Geometry: final body of the model. Coordinates: model frame, mm. A direction names the side the tool comes from. Round coordinates to 2 decimals unless told otherwise and drop trailing zeros. Write each loop counter-clockwise with the first axis right and the second up, starting at its lowest first coordinate (ties: lowest second). Pieces come first, ordered by that corner, then holes. Notation, with made-up numbers: M -2,-37 L 10,-37 A31 ccw 10,-8 Z; hole C 27.5,-37 d8. An arc over 180 degrees is marked long. Answer as CSV lines item,"result". Start each with the question number.
Q1. Section query A-A on z = 234. Output: boundary loops of the cut face in (x, y).
Q2. Section query C-C on y = 6. Output: boundary loops of the cut face in (x, z), and give its area (3 significant figures).
Q3. Mould query, pull axis Z, two halves, no side actions, for faces 1 (the flat face through (-151.164, -3, 200)), 2 (the flat face through (-40.966, -20.171, 17.605)), 3 (the flat face through (-110, -3, 147.99)), 4 (the flat face through (-151.164, -3, 277)). Classes: pulls with the +Z half, pulls with the -Z half, needs draft (parallel to the pull), parting line crosses it, or undercut.
Q4. First-contact query: pin 1 (4 mm diameter, centred on x = -59, y = -1, fed in from +Z); pin 2 (5 mm diameter, centred on x = -195, y = -4.5, fed in from -Z); pin 3 (12 mm diameter, centred on y = -10.5, z = 121.5, fed in from +X). Flat tips, straight axial feed; report the tip coordinate or a pass-through.
Q5. Reachability of faces 5 (the flat face through (-13.889, -5, 132)), 6 (the flat face through (-220.841, -3, 248)), 7 (the flat face through (-109, -3, 137.605)), 8 (the flat face through (-157, -8, 206)) from +Z, -Z, +X, -X, +Y, -Y: full face, straight path, thin tool, end or side. Return the list, or none.
Q6. Section query B-B on x = -89. Output: boundary loops of the cut face in (y, z).
Q7. Ray query, probe 1 along Z at (x, y) = (-183, -6); probe 2 along X at (y, z) = (1, 270.5); probe 3 along X at (y, z) = (-6, 216). Return the intervals inside material, ascending.
Q8. Section query D-D on z = 92.5. Output: boundary loops of the cut face in (x, y).
```python
from build123d import *

# Parameters (mm, degrees)
SKETCH_1_W      = 68.292893219
SKETCH_1_H      = 68.292893218
EXTRUDE_1_DEPTH = 10
SKETCH_2_W      = 53.40749746
SKETCH_2_H      = 14.776374923
EXTRUDE_2_DEPTH = 270
SKETCH_4_W      = 27.47748939
SKETCH_4_H      = 82.93676663
SKETCH_4_H_2    = 74.09911356
SKETCH_4_W_2    = 31.70911111
EXTRUDE_3_DEPTH = 10
CHAMFER_1_SIZE  = 15
CHAMFER_3_SIZE  = 7
FILLET_3_R      = 5
CHAMFER_4_SIZE  = 4


with BuildPart() as part:
    # 草图1 → 凸台-拉伸1 (new body)
    with BuildSketch(Plane.XY):
        with Locations((-33.149855831, 2)):
            Rectangle(SKETCH_1_W, SKETCH_1_H)
    extrude(amount=EXTRUDE_1_DEPTH)

    # 草图2 → 凸台-拉伸2 (add)
    with BuildSketch(Plane.XY.offset(10)):
        with Locations((-40.59255371, -5.388187462)):
            Rectangle(SKETCH_2_W, SKETCH_2_H)
    extrude(amount=EXTRUDE_2_DEPTH)

    # 草图4 → 凸台-拉伸3 (add)
    with BuildSketch(Plane(origin=(0, 2, 0), x_dir=(1, 0, 0), z_dir=(0, 1, 0))):
        Polygon((-151.163737931, -260.803324395), (-67.29630244, -260.803324395), (-67.29630244, -249.935229756), (-151.163737931, -249.935229756), (-151.163737931, -147.989777894), (-67.29630244, -147.989777894), (-67.29630244, -137.604662475), (-151.163737931, -137.604662475), (-151.163737931, -117.751683705), (-229.082858204, -117.751683705), (-229.082858204, -294.217578605), (-151.163737931, -294.217578605), align=None)
        with Locations((-207.102608026, -247.45301447)):
            Rectangle(SKETCH_4_W, SKETCH_4_H, mode=Mode.SUBTRACT)
        with Locations((-207.102608026, -162.803209554)):
            Rectangle(SKETCH_4_W, SKETCH_4_H_2, mode=Mode.SUBTRACT)
        with Locations((-172.622136648, -247.45301447)):
            Rectangle(SKETCH_4_W_2, SKETCH_4_H, mode=Mode.SUBTRACT)
        with Locations((-172.622136648, -162.803209554)):
            Rectangle(SKETCH_4_W_2, SKETCH_4_H_2, mode=Mode.SUBTRACT)
    extrude(amount=-EXTRUDE_3_DEPTH)

    # 倒角1
    chamfer_1_edges = [part.edges().sort_by_distance(p)[0] for p in [
        (-40.59255371, 2, 10),
        (-40.59255371, -12.776374923, 10),
    ]]
    chamfer(chamfer_1_edges, length=CHAMFER_1_SIZE)

    # 倒角3
    chamfer_3_edges = [part.edges().sort_by_distance(p)[0] for p in [
        (-229.082858204, -8, 205.984631155),
    ]]
    chamfer(chamfer_3_edges, length=CHAMFER_3_SIZE)

    # 圆角3
    fillet_3_edges = [part.edges().sort_by_distance(p)[0] for p in [
        (-13.88880498, -5.388187462, 280),
        (-67.29630244, -5.388187462, 280),
        (-220.841352721, -3, 125.753652774),
        (-220.841352721, -3, 205.984631155),
        (-193.363863331, -3, 288.921397785),
        (-220.841352721, -3, 288.921397785),
        (-156.767581093, -3, 288.921397785),
        (-156.767581093, -3, 199.852766334),
        (-188.476692203, -3, 125.753652774),
        (-156.767581093, -3, 125.753652774),
        (-193.363863331, -3, 125.753652774),
        (-151.163737931, -3, 294.217578605),
        (-151.163737931, -3, 117.751683705),
        (-193.363863331, -3, 199.852766334),
        (-156.767581093, -3, 205.984631155),
        (-193.363863331, -3, 205.984631155),
        (-220.841352721, -3, 199.852766334),
        (-188.476692203, -3, 199.852766334),
        (-188.476692203, -3, 205.984631155),
        (-188.476692203, -3, 288.921397785),
    ]]
    fillet(fillet_3_edges, radius=FILLET_3_R)

    # 倒角4
    chamfer_4_edges = [part.edges().sort_by_distance(p)[0] for p in [
        (-67.29630244, -3, 249.935229756),
        (-67.29630244, -3, 260.803324395),
        (-151.163737931, -3, 260.803324395),
        (-151.163737931, -3, 137.604662475),
        (-67.29630244, -3, 137.604662475),
        (-67.29630244, -3, 147.989777894),
        (-151.163737931, -3, 147.989777894),
        (-151.163737931, -3, 249.935229756),
    ]]
    chamfer(chamfer_4_edges, length=CHAMFER_4_SIZE)


solid = part.part
```
Entries:
1,outline,"M -229.08,-1 L -222.08,-8 L -220.84,-8 L -220.84,2 L -229.08,2 Z; M -193.36,-8 L -188.48,-8 L -188.48,2 L -193.36,2 Z; M -156.77,-8 L -151.16,-8 L -151.16,2 L -156.77,2 Z; M -67.3,-12.78 L -13.89,-12.78 L -13.89,2 L -67.3,2 Z"
2,outline,"M -67.3,0 L 1,0 L 1,10 L -13.89,10 L -13.89,21 L -67.3,21 Z"
2,area,"1,270 mm^2"
3,face 1,"undercut"
3,face 2,"pulls with the +Z half"
3,face 3,"undercut"
3,face 4,"needs draft"
4,pin 1,"stops at z = 280"
4,pin 2,"stops at z = 117.75"
4,pin 3,"stops at x = -13.89"
5,face 5,"+Z, +X, +Y, -Y"
5,face 6,"+Y, -Y"
5,face 7,"-Z, +Y, -Y"
5,face 8,"+Z, -Z, -X, -Y"
6,outline,"M -8,137.6 L 2,137.6 L 2,147.99 L -8,147.99 Z; M -8,249.94 L 2,249.94 L 2,260.8 L -8,260.8 Z"
7,probe 1,"z = 117.75 to 125.75, 199.85 to 205.98, 288.92 to 294.22"
7,probe 2,"x = -229.08 to -220.84, -193.36 to -188.48, -156.77 to -151.16, -67.3 to -13.89"
7,probe 3,"x = -224.08 to -220.84, -193.36 to -188.48, -156.77 to -151.16, -67.3 to -13.89"
8,outline,"M -67.3,-12.78 L -13.89,-12.78 L -13.89,2 L -67.3,2 Z"
